Here's how the part is built. I have some questions about the finished solid (model axes, mm). A direction names the side the tool comes from. Coordinates: 2 decimals unless noted, no trailing zeros. Write each loop counter-clockwise with the first axis right and the second up, starting at its lowest first coordinate (ties: lowest second). Pieces come first, ordered by that corner, then holes.
from build123d import *

# Parameters (mm, degrees)
F1_R     = 19.05
F2_DEPTH = 1778
F4_DEPTH = 25.4
F5_W     = 152.4
F5_H     = 152.4
F6_DEPTH = 25.4


with BuildPart() as f2:
    # F1 (on face) → F2 (new body)
    with BuildSketch(Plane.XZ):
        with BuildLine():
            ThreePointArc((808.430407, 0), (884.630407, 76.2), (808.430407, 152.4))
            Line((808.430407, 152.4), (-105.969593, 152.4))
            ThreePointArc((-105.969593, 152.4), (-182.169593, 76.2), (-105.969593, 0))
            Line((-105.969593, 0), (808.430407, 0))
        make_face()
        with Locations((-106.129967, 76.004088)):
            Circle(F1_R, mode=Mode.SUBTRACT)
        with Locations((807.696342, 75.448431)):
            Circle(F1_R, mode=Mode.SUBTRACT)
    extrude(amount=F2_DEPTH)

    # F3 (on face) → F4 (join)
    with BuildSketch(Plane.XZ.offset(1778)):
        Polygon((427.430407, 152.4), (351.230407, 152.4), (275.030407, 152.4), (275.030407, 0), (427.430407, 0), align=None)
    extrude(amount=F4_DEPTH)

    # F5 (on face) → F6 (join)
    with BuildSketch(Plane.XZ):
        with Locations((351.230407, 76.2)):
            Rectangle(F5_W, F5_H)
    extrude(amount=-F6_DEPTH)


solid = f2.part
1. I want a section at B-B (z = 32.5). List the corners of the cut face in (x, y) for me, then the cut area to 3 significant figures.
2. On a 3-axis mill with a long thin cutter (end or side, diameter ignored), from which of +Z, -Z, +X, -X, +Y, -Y can I reach the whole of each face in a straight line? I mean faces 1 (the face through (43, -1778, 77)), 2 (the face through (653, -1778, 77)), 3 (the face through (43, 0, 77)). Say none if no direction works.
3. If I drill on line 1 (X direction, y = -265, z = 60); line 2 (Y direction, x = 589, z = 15.5); line 3 (X direction, y = -347.5, z = 63.5), over which ranges is the centre line in solid material (lowest first)?
4. I want a section at C-C (x = 596.5). List the corners of the cut face in (y, z) for me, then the cut area to 3 significant figures.
5. I want a section at A-A (y = -372). List the corners of the cut face in (x, z) for me.
6. For pin 1 Ø12 at (y, z) = (-894, 84.5) entering from +X; pin 2 Ø7.5 at (y, z) = (-1790, 68) entering from -X; pin 3 Ø12 at (y, z) = (-674.5, 26) entering from -X, each with a flat end and sliding along its axis, tell me the tip position at first contact or that it passes through.
7. Thinking about a two-plate mould opening in X: for faces 4 (the face through (358, -876, 152.4)), 5 (the face through (-97.34, -876.554, 59.103)), 6 (the face through (825.867, -876.554, 81.171)), 7 (the face through (884.61, -876.55, 74.52)), which applies, pulls with the +X half, pulls with the -X half, needs draft (parallel to the pull), parting line crosses it, or undercut?
Response values:
1. outline: (-168.39, -1778) - (275.03, -1778) - (275.03, -1803.4) - (427.43, -1803.4) - (427.43, -1778) - (870.85, -1778) - (870.85, 0) - (427.43, 0) - (427.43, 25.4) - (275.03, 25.4) - (275.03, 0) - (-168.39, 0) - close
1. area: 1,860,000 mm2
2. face 1: +Z, -Z, -X, -Y
2. face 2: +Z, -Z, +X, -Y
2. face 3: +Z, -Z, -X, +Y
3. line 1: x = -180.43 to -116.46, -95.8 to 796.55, 818.84 to 882.89
3. line 2: y = -1778 to 0
3. line 3: x = -181.1 to -120.5, -91.76 to 792.86, 822.53 to 883.56
4. outline: (-1778, 0) - (0, 0) - (0, 152.4) - (-1778, 152.4) - close
4. area: 271,000 mm2
5. outline: (-105.97, 0) - (808.43, 0) arc R76.2 ccw to (808.43, 152.4) - (-105.97, 152.4) arc R76.2 ccw to start; hole circle Ø38.1 at (-106.13, 76); hole circle Ø38.1 at (807.7, 75.45)
6. pin 1: stops at x = 884.6
6. pin 2: stops at x = 275.03
6. pin 3: stops at x = -168.04
7. face 4: needs draft
7. face 5: undercut
7. face 6: undercut
7. face 7: pulls with the +X half
